Autodesk Inventor part; units mm, degrees
ref_plane "YZ Plane" through (0, 0, 0) normal (1, 0, 0) x (0, 1, 0)
ref_plane "XZ Plane" through (0, 0, 0) normal (0, 1, 0) x (-1, 0, 0)
ref_plane "XY Plane" through (0, 0, 0) normal (0, 0, 1) x (1, 0, 0)
sketch "Sketch1" plane through (0, 0, 0) normal (0, 0, 1) x (1, 0, 0)
  circle A0 centre (0, 0) radius 22.775
  dimension "d0" = 45.55
extrude "Extrusion1" add sketch "Sketch1" along normal blind 5.78
sketch "Sketch2" plane through (0, 0, 5.78) normal (0, 0, 1) x (1, 0, 0)
  circle A0 centre (0, 0) radius 18
  dimension "d3" = 36
extrude "Through-hole" cut sketch "Sketch2" against normal blind 548
sketch "Sketch3" plane through (0, 0, 5.78) normal (0, 0, 1) x (1, 0, 0)
  circle A0 centre (0, 0) radius 20.25
  dimension "d6" = 40.5
extrude "snug ring fit" cut sketch "Sketch3" against normal blind 5
sketch "Sketch4" plane through (0, 0, 0) normal (0, 1, 0) x (-1, 0, 0)
  line L0 (22.775, 5.78) -> (-22.775, 5.78)
  line L1 (0, 5.78) -> (0, 3.78)
  circle A0 centre (0, 3.78) radius 1
  point P0 (0, 0)
  dimension "d9" = 2
  dimension "d10" = 2
extrude "Extrusion4" cut sketch "Sketch4" along normal mid plane 548
properties part number "Diaphragm_lock"
Build history of the part. All positions in model axes, mm. A direction names the side the tool comes from. Round coordinates to 2 decimals unless told otherwise and drop trailing zeros. Write each loop counter-clockwise with the first axis right and the second up, starting at its lowest first coordinate (ties: lowest second). Pieces come first, ordered by that corner, then holes. Notation, with made-up numbers: (11.5, 52) -> (58.5, 52) arc R30 ccw to (58.5, 88) -> close; hole circle Ø4 at (-23, 47). An arc over 180 degrees is marked (long way). Use one line per item in the form item = value.
Q1. Two-plate mould, pull along Z, no slides. Class faces 3 (the cylindrical face through (-2.343, 17.847, 0.395)), 4 (the flat face through (17, 7, 0)), 5 (the cylindrical face through (0.2, -21.5, 2.8)): released by +Z, released by -Z, zero draft, split by the parting line, or undercut.
Conclusion:
face_3 = zero draft
face_4 = released by -Z
face_5 = undercut
Q2. Drill centre lines: L1, parallel to Z at x = 0, y = -21; L2, parallel to Y at x = 11.5, z = 5.1; L3, parallel to X at y = -2.5, z = 2.25. Where is each one in solid material? Low to high.
Conclusion:
L1 = 0 to 2.78, 4.78 to 5.78
L2 = -19.66 to -16.67, 16.67 to 19.66
L3 = -22.64 to -20.1, 20.1 to 22.64
Q3. Band-saw the part on C-C, the plane x = 12. Write the cut outline in (y, z), then the cut area to 3 significant figures.
Conclusion:
outline = (-19.36, 0) -> (-13.42, 0) -> (-13.42, 0.78) -> (-16.31, 0.78) -> (-16.31, 5.78) -> (-19.36, 5.78) -> close; (13.42, 0) -> (19.36, 0) -> (19.36, 5.78) -> (16.31, 5.78) -> (16.31, 0.78) -> (13.42, 0.78) -> close
area = 39.7 mm²
Q4. Tool access for faces 1 (the cylindrical face through (-0.46, 21.48, 4.67)), 2 (the cylindrical face through (11, 17, 3)): list every direction of +Z, -Z, +X, -X, +Y, -Y with a clear straight run to the whole face (end or side of a thin tool).
Conclusion:
face_1 = +Y, -Y
face_2 = +Z
Q5. Drop flat-ended pins along their axis: P1, Ø1.8, axis at x = 0, z = 3.78, coming from the +Y side; P2, Ø2, axis at y = 12, z = 3, coming from the -X side; P3, Ø2, axis at y = -13, z = 2, coming from the -X side; P4, Ø3, axis at y = 8.5, z = 2, coming from the +X side. Give the stop position or say it passes through.
Conclusion:
P1 = through
P2 = -19.94
P3 = -19.36
P4 = 21.67
Q6. Band-saw the part on A-A, the plane y = 0. Write the cut outline in (x, z) (3 decimals), then the cut area to 3 significant figures.
Conclusion:
outline = (-22.775, 0) -> (-18, 0) -> (-18, 0.78) -> (-20.25, 0.78) -> (-20.25, 5.78) -> (-22.775, 5.78) -> close; (18, 0) -> (22.775, 0) -> (22.775, 5.78) -> (20.25, 5.78) -> (20.25, 0.78) -> (18, 0.78) -> close
area = 32.7 mm²
Q7. Band-saw the part on B-B, the plane x = 0. Write the cut outline in (y, z) (3 decimals), then the cut area to 3 significant figures.
Conclusion:
outline = (-22.775, 0) -> (-18, 0) -> (-18, 0.78) -> (-20.25, 0.78) -> (-20.25, 2.78) -> (-22.775, 2.78) -> close; (-22.775, 4.78) -> (-20.25, 4.78) -> (-20.25, 5.78) -> (-22.775, 5.78) -> close; (18, 0) -> (22.775, 0) -> (22.775, 2.78) -> (20.25, 2.78) -> (20.25, 0.78) -> (18, 0.78) -> close; (20.25, 4.78) -> (22.775, 4.78) -> (22.775, 5.78) -> (20.25, 5.78) -> close
area = 22.6 mm²
Q8. Band-saw the part on D-D, the plane z = 3.78. Write the cut outline in (x, y) (3 decimals).
Conclusion:
outline = (-1, -22.753) -> (-1, -20.225) arc R20.25 cw to (-1, 20.225) -> (-1, 22.753) arc R22.775 ccw to start; (1, -22.753) arc R22.775 ccw to (1, 22.753) -> (1, 20.225) arc R20.25 cw to (1, -20.225) -> close
